Check sheet for the modelled part. Datum: model origin and axes. Units: mm. Give positions to 0.01 mm unless a question says otherwise; leave off trailing zeros. Write each loop counter-clockwise with the first axis right and the second up, starting at its lowest first coordinate (ties: lowest second). Pieces come first, ordered by that corner, then holes. Notation, with made-up numbers: M 55,-7 L 75,-7 A21 ccw 75,8 Z; hole C 54.25,44 d7. An arc over 180 degrees is marked long. Write each question's results on one line, items separated by ' | '. Start each with the question number.
from build123d import *

# Parameters (mm, degrees)
SKETCH1_R           = 5
SKETCH1_R_2         = 2.5
BOSS_EXTRUDE1_DEPTH = 4.7
CHAMFER1_SIZE       = 1
CHAMFER1_SIZE2      = 0.577350269
CHAMFER2_SIZE       = 1
CHAMFER2_SIZE2      = 0.577350269
SKETCH1_3_R         = 5
CUT_EXTRUDE1_DEPTH  = 9.490583019
CHAMFER3_SIZE       = 0.5


with BuildPart() as part:
    # Sketch1 → Boss-Extrude1 (new body)
    # profile 1 of 2: a face of its own
    with BuildSketch(Plane.XY):
        Circle(SKETCH1_R)
        Polygon((4, 2.309401077), (0, 4.618802154), (-4, 2.309401077), (-4, -2.309401077), (0, -4.618802154), (4, -2.309401077), align=None, mode=Mode.SUBTRACT)
    # profile 2 of 2: a face of its own
    with BuildSketch(Plane.XY):
        Polygon((4, -2.309401077), (4, 2.309401077), (0, 4.618802154), (-4, 2.309401077), (-4, -2.309401077), (0, -4.618802154), align=None)
        Circle(SKETCH1_R_2, mode=Mode.SUBTRACT)
    extrude(amount=BOSS_EXTRUDE1_DEPTH)

    # Chamfer1
    chamfer1_edges = [part.edges().sort_by_distance(p)[0] for p in [
        (-5, 0, 4.7),
    ]]
    chamfer1_side = [part.faces().sort_by_distance(p)[0] for p in [
        (-4.858578644, 0, 4.7),
    ]]
    chamfer(chamfer1_edges, length=CHAMFER1_SIZE, length2=CHAMFER1_SIZE2, reference=chamfer1_side[0])

    # Chamfer2
    chamfer2_edges = [part.edges().sort_by_distance(p)[0] for p in [
        (-5, 0, 0),
    ]]
    chamfer2_side = [part.faces().sort_by_distance(p)[0] for p in [
        (-4.858578644, 0, 0),
    ]]
    chamfer(chamfer2_edges, length=CHAMFER2_SIZE, length2=CHAMFER2_SIZE2, reference=chamfer2_side[0])

    # Sketch1_3 → Cut-Extrude1 (cut, through all)
    with BuildSketch(Plane.XY):
        Circle(SKETCH1_3_R)
        Polygon((4, 2.309401077), (0, 4.618802154), (-4, 2.309401077), (-4, -2.309401077), (0, -4.618802154), (4, -2.309401077), align=None, mode=Mode.SUBTRACT)
    extrude(amount=CUT_EXTRUDE1_DEPTH, mode=Mode.SUBTRACT)

    # Chamfer3
    chamfer3_edges = [part.edges().sort_by_distance(p)[0] for p in [
        (-2.5, 0, 0),
        (-2.5, 0, 4.7),
    ]]
    chamfer(chamfer3_edges, length=CHAMFER3_SIZE)


solid = part.part
Q1. Section check A-A on z = 1.2. Record the boundary of the cut face in (x, y), plus the area to 3 significant figures.
Q2. Release check for a two-part mould opening along X. For faces 1 (the face through (3.589, -2.084, 4.613)), 2 (the face through (1, 3, 4.7)), 3 (the face through (-0.54, -2.44, 2.32)) record: pulls with the +X half, pulls with the -X half, needs draft (parallel to the pull), parting line crosses it, or undercut.
Q3. Depth check by flat-ended pin: pin 1 Ø4.5 at (x, y) = (0, 0) entering from -Z. Enter the tip coordinate at first touch or a pass-through.
Q4. Scan lines: L1, parallel to Y at x = -1, z = 3.2; L2, parallel to Y at x = -1.5, z = 2; L3, parallel to X at y = -0.25, z = 0.7. Record each from-to range of solid material in increasing order.
Check result:
1) outline: M -4,-2.31 L 0,-4.62 L 4,-2.31 L 4,2.31 L 0,4.62 L -4,2.31 Z; hole C 0,0 d5 | area: 35.8 mm^2
2) face 1: pulls with the +X half | face 2: needs draft | face 3: undercut
3) pin 1: through
4) L1: -4.04 to -2.29, 2.29 to 4.04 | L2: -3.75 to -2, 2 to 3.75 | L3: -4 to -2.49, 2.49 to 4
